from build123d import *

# Parameters (mm, degrees)
F0_R     = 2.9972
F0_R_2   = 1.016
F0_W     = 42.0375
F0_H     = 10.9479
F1_DEPTH = 2.54
F3_D     = 2.032
F4_R     = 1.5875


with BuildPart() as f1:
    # F0 (on Front) → F1 (new body)
    with BuildSketch(Plane.XZ):
        with BuildLine():
            ThreePointArc((-76.2, 5.88645), (-82.08645, 0), (-76.2, -5.88645))
            Line((-76.2, -5.88645), (-28.575, -5.88645))
            Line((-28.575, -5.88645), (-28.575, -13.0302))
            Line((-28.575, -13.0302), (28.575, -13.0302))
            Line((28.575, -13.0302), (28.575, -5.88645))
            Line((28.575, -5.88645), (76.2, -5.88645))
            ThreePointArc((76.2, -5.88645), (82.08645, 0), (76.2, 5.88645))
            Line((76.2, 5.88645), (28.575, 5.88645))
            Line((28.575, 5.88645), (28.575, 13.0302))
            Line((28.575, 13.0302), (-28.575, 13.0302))
            Line((-28.575, 13.0302), (-28.575, 5.88645))
            Line((-28.575, 5.88645), (-76.2, 5.88645))
        make_face()
        with Locations((-76.2, 0)):
            Circle(F0_R, mode=Mode.SUBTRACT)
        with Locations((-63.5, 0)):
            Circle(F0_R_2, mode=Mode.SUBTRACT)
        with BuildLine():
            Line((-70.5263540646, -1.56845), (-34.417, -1.56845))
            Line((-34.417, -1.56845), (-28.575, -1.56845))
            Line((-28.575, -1.56845), (-28.575, -3.34645))
            Line((-28.575, -3.34645), (-71.3573183049, -3.34645))
            ThreePointArc((-71.3573183049, -3.34645), (-70.8672138888, -2.492325399), (-70.5263540646, -1.56845))
        make_face(mode=Mode.SUBTRACT)
        with BuildLine():
            ThreePointArc((-55.753, 0), (-54.737, 1.016), (-53.721, 0))
            ThreePointArc((-53.721, 0), (-54.737, -1.016), (-55.753, 0))
        make_face(mode=Mode.SUBTRACT)
        with BuildLine():
            ThreePointArc((-50.673, 0), (-49.657, 1.016), (-48.641, 0))
            ThreePointArc((-48.641, 0), (-49.657, -1.016), (-50.673, 0))
        make_face(mode=Mode.SUBTRACT)
        with BuildLine():
            ThreePointArc((-45.593, 0), (-44.577, 1.016), (-43.561, 0))
            ThreePointArc((-43.561, 0), (-44.577, -1.016), (-45.593, 0))
        make_face(mode=Mode.SUBTRACT)
        with BuildLine():
            ThreePointArc((-40.513, 0), (-39.497, 1.016), (-38.481, 0))
            ThreePointArc((-38.481, 0), (-39.497, -1.016), (-40.513, 0))
        make_face(mode=Mode.SUBTRACT)
        with BuildLine():
            ThreePointArc((-35.433, 0), (-35.1354204897, 0.7184204897), (-34.417, 1.016))
            ThreePointArc((-34.417, 1.016), (-33.6985795103, 0.7184204897), (-33.401, 0))
            ThreePointArc((-33.401, 0), (-33.6985795103, -0.7184204897), (-34.417, -1.016))
            ThreePointArc((-34.417, -1.016), (-35.1354204897, -0.7184204897), (-35.433, 0))
        make_face(mode=Mode.SUBTRACT)
        Rectangle(F0_W, F0_H, mode=Mode.SUBTRACT)
        with BuildLine():
            Line((28.575, -2.71145), (28.575, 2.71145))
            Line((28.575, 2.71145), (56.2761407595, 2.71145))
            Line((56.2761407595, 2.71145), (59.3600312801, 0.1745531584))
            ThreePointArc((59.3600312801, 0.1745531584), (59.3563530789, 0), (59.3600312801, -0.1745531584))
            Line((59.3600312801, -0.1745531584), (56.2761407595, -2.71145))
            Line((56.2761407595, -2.71145), (28.575, -2.71145))
        make_face(mode=Mode.SUBTRACT)
        with BuildLine():
            Line((58.2752193826, -2.71145), (59.6646676279, -1.56845))
            Line((59.6646676279, -1.56845), (70.5263540646, -1.56845))
            ThreePointArc((70.5263540646, -1.56845), (70.8672138888, -2.492325399), (71.3573183049, -3.34645))
            Line((71.3573183049, -3.34645), (58.6573183049, -3.34645))
            ThreePointArc((58.6573183049, -3.34645), (58.4562657085, -3.0349691924), (58.2752193826, -2.71145))
        make_face(mode=Mode.SUBTRACT)
        with Locations((63.5, 0)):
            Circle(F0_R_2, mode=Mode.SUBTRACT)
        with Locations((76.2, 0)):
            Circle(F0_R, mode=Mode.SUBTRACT)
        with BuildLine():
            Line((-28.575, 1.56845), (-34.417, 1.56845))
            Line((-34.417, 1.56845), (-70.5263540646, 1.56845))
            ThreePointArc((-70.5263540646, 1.56845), (-70.8672138888, 2.492325399), (-71.3573183049, 3.34645))
            Line((-71.3573183049, 3.34645), (-28.575, 3.34645))
            Line((-28.575, 3.34645), (-28.575, 1.56845))
        make_face(mode=Mode.SUBTRACT)
        with BuildLine():
            ThreePointArc((58.2752193826, 2.71145), (58.4562657085, 3.0349691924), (58.6573183049, 3.34645))
            Line((58.6573183049, 3.34645), (71.3573183049, 3.34645))
            ThreePointArc((71.3573183049, 3.34645), (70.8672138888, 2.492325399), (70.5263540646, 1.56845))
            Line((70.5263540646, 1.56845), (59.6646676279, 1.56845))
            Line((59.6646676279, 1.56845), (58.2752193826, 2.71145))
        make_face(mode=Mode.SUBTRACT)
    extrude(amount=-F1_DEPTH)

    # F3 (through all)
    with Locations(Plane.XZ):
        with Locations((-23.01875, 7.47395), (-18.25625, 7.47395), (-13.49375, 7.47395), (-8.73125, 7.47395), (-3.96875, 7.47395), (-0.00635, 7.47395), (3.96875, 7.47395), (8.73125, 7.47395), (13.49375, 7.47395), (18.25625, 7.47395), (23.0101440102, 7.47395), (23.01875, -3.1105038886), (23.01875, -7.47395), (23.01875, 2.71145), (18.25625, -7.47395), (13.49375, -7.47395), (8.73125, -7.47395), (3.96875, -7.47395), (-0.00635, -7.47395), (-3.96875, -7.47395), (-8.73125, -7.47395), (-13.49375, -7.47395), (-18.25625, -7.47395), (-23.01875, -7.47395), (-23.01875, -2.71145), (-23.01875, 2.71145)):
            Hole(F3_D / 2)

    # F4
    f4_edges = [f1.edges().sort_by_distance(p)[0] for p in [
        (-34.417, 1.27, 1.016),
        (-28.575, 1.27, 13.0302),
        (-28.575, 1.27, 5.88645),
        (-28.575, 1.27, -13.0302),
        (-28.575, 1.27, -5.88645),
        (28.575, 1.27, 2.71145),
        (28.575, 1.27, 13.0302),
        (28.575, 1.27, -5.88645),
        (28.575, 1.27, -13.0302),
        (28.575, 1.27, 5.88645),
        (28.575, 1.27, -2.71145),
    ]]
    fillet(f4_edges, radius=F4_R)


solid = f1.part
Verification items for the finished model (mm, model axes). A direction names the side the tool comes from. Round coordinates to 2 decimals unless told otherwise and drop trailing zeros. Answer in a Markdown table with one row per item. Add a question column.
Q1. Gauge pin test, flat ends, axial feed: pin 1 (1.2 mm diameter, centred on x = 8.73, z = 7.47, fed in from +Y); pin 2 (0.8 mm diameter, centred on x = 65.5, y = 1, fed in from +Z). Record the tip position at first contact, or that the pin passes through.
Q2. Tool access check on faces 1 (the face through (-28.575, 1, 9)), 2 (the face through (28.575, 1, -9)), 3 (the face through (54, 1, 5.886)), 4 (the face through (43, 1, 2.711)), 5 (the face through (-54, 1, -5.886)). Record the directions out of +Z, -Z, +X, -X, +Y, -Y that give a thin tool (end or side, any length) a straight path to the whole face; none if there is none.
Q3. Release check for a two-part mould opening along Z. For faces 6 (the face through (-50, 1, -3.346)), 7 (the face through (-53, 1, 5.886)), 8 (the face through (53, 1, -5.886)), 9 (the face through (82.085, 1.252, -0.129)) record: pulls with the +Z half, pulls with the -Z half, needs draft (parallel to the pull), parting line crosses it, or undercut.
Q4. Section check A-A on y = 2.1. State how many separate pieces and enclosed holes the cut face has, plus the area to 3 significant figures.
Q5. Material ranges on line 1 (Z direction, x = -68, y = 2.25); line 2 (Z direction, x = -63.5, y = 1.85); line 3 (Z direction, x = 16, y = 1.2), recorded low to high.
Found:
| question | item | result |
|---|---|---|
| 1 | pin 1 | passes through |
| 1 | pin 2 | stops at z = 5.89 |
| 2 | face 1 | +Z, -X, +Y, -Y |
| 2 | face 2 | -Z, +X, +Y, -Y |
| 2 | face 3 | +Z, +X, +Y, -Y |
| 2 | face 4 | +Y, -Y |
| 2 | face 5 | -Z, -X, +Y, -Y |
| 3 | face 6 | undercut |
| 3 | face 7 | pulls with the +Z half |
| 3 | face 8 | pulls with the -Z half |
| 3 | face 9 | parting line crosses it |
| 4 | separate pieces | 1 |
| 4 | enclosed holes | 41 |
| 4 | area | 1,740 mm² |
| 5 | line 1 | z = -5.89 to -3.35, -1.57 to 1.57, 3.35 to 5.89 |
| 5 | line 2 | z = -5.89 to -3.35, -1.57 to -1.02, 1.02 to 1.57, 3.35 to 5.89 |
| 5 | line 3 | z = -13.03 to -5.47, 5.47 to 13.03 |
